Print and shaded views of the part. All mm, measured from the part's lowest x, y and z. A direction names the side the tool comes from. Round coordinates to 2 decimals unless told otherwise and drop trailing zeros. Write each loop counter-clockwise with the first axis right and the second up, starting at its lowest first coordinate (ties: lowest second). Pieces come first, ordered by that corner, then holes. Notation, with made-up numbers: M 64,7.5 L 115,7.5 A21 ccw 115,20.5 Z; hole C -19,13 d3. An arc over 180 degrees is marked long. Write item = value, one per line.
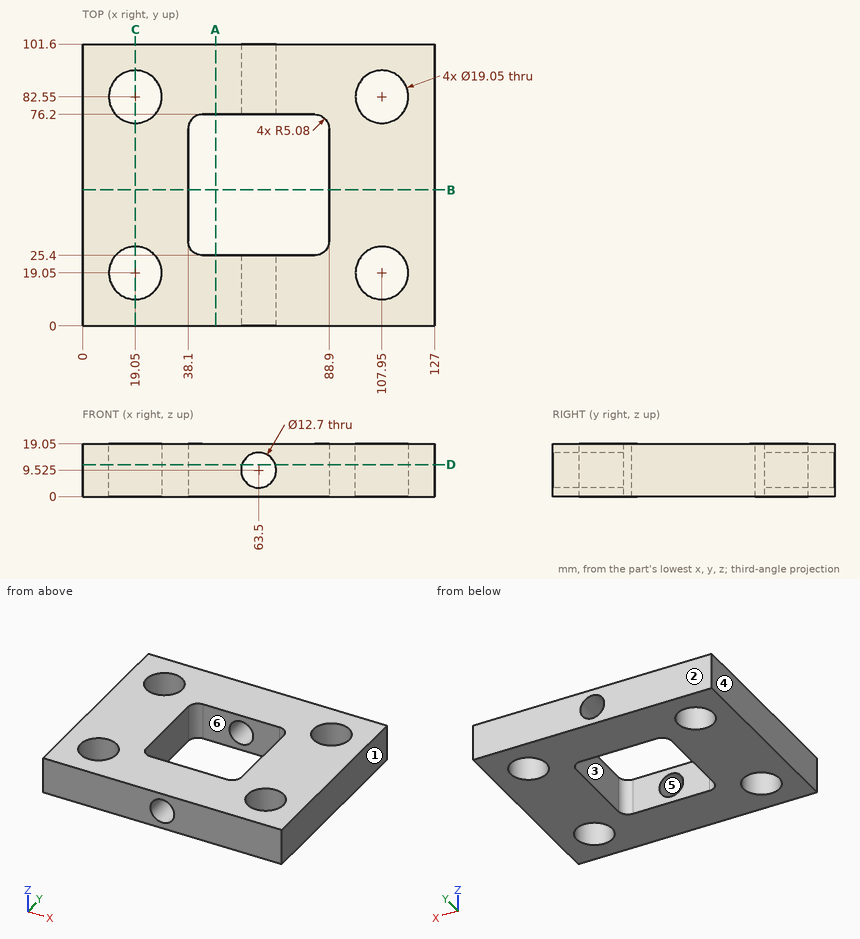
1. Flat gauge pin, fed straight in: pin 1 (17 mm diameter, centred on x = 107.95, y = 19.05, fed in from -Z). Where does the tip first touch, or does it go through?
Responses:
pin_1 = through
2. Band-saw the part on D-D (z = 11.5). List the corners of the cut face in (x, y) (3 decimals).
Responses:
outline = M 0,0 L 57.465,0 L 57.465,25.4 L 43.18,25.4 A5.08 cw 38.1,30.48 L 38.1,71.12 A5.08 cw 43.18,76.2 L 57.465,76.2 L 57.465,101.6 L 0,101.6 Z; M 69.535,0 L 127,0 L 127,101.6 L 69.535,101.6 L 69.535,76.2 L 83.82,76.2 A5.08 cw 88.9,71.12 L 88.9,30.48 A5.08 cw 83.82,25.4 L 69.535,25.4 Z; hole C 19.05,19.05 d19.05; hole C 19.05,82.55 d19.05; hole C 107.95,19.05 d19.05; hole C 107.95,82.55 d19.05
3. Mould opens along X. For the marked faces 1, 2, 3 and 4 say: pulls with the +X half, pulls with the -X half, needs draft (parallel to the pull), parting line crosses it, or undercut.
Responses:
face_1 = pulls with the +X half
face_2 = needs draft
face_3 = undercut
face_4 = pulls with the -X half
4. Band-saw the part on C-C (x = 19.05). List the corners of the cut face in (y, z) (3 decimals).
Responses:
outline = M 0,0 L 9.525,0 L 9.525,19.05 L 0,19.05 Z; M 28.575,0 L 73.025,0 L 73.025,19.05 L 28.575,19.05 Z; M 92.075,0 L 101.6,0 L 101.6,19.05 L 92.075,19.05 Z
5. Probe probe 1 along Y at (x, z) = (19.05, 4.75) (3 decimals); probe 2 along Y at (x, z) = (25, 7.5); probe 3 along X at (y, z) = (31.5, 9.75). List the from-to ranges inside material, lowest first.
Responses:
probe_1 = 0 to 9.525, 28.575 to 73.025, 92.075 to 101.6
probe_2 = 0 to 11.61, 26.49 to 75.11, 89.99 to 101.6
probe_3 = 0 to 38.1, 88.9 to 127
6. Tool access for the marked faces 5 and 6: list every direction of +Z, -Z, +X, -X, +Y, -Y with a clear straight run to the whole face (end or side of a thin tool).
Responses:
face_5 = +Y, -Y
face_6 = +Z, -Z
7. Band-saw the part on B-B (y = 49). List the corners of the cut face in (x, z).
Responses:
outline = M 0,0 L 38.1,0 L 38.1,19.05 L 0,19.05 Z; M 88.9,0 L 127,0 L 127,19.05 L 88.9,19.05 Z
8. Band-saw the part on A-A (x = 48). List the corners of the cut face in (y, z).
Responses:
outline = M 0,0 L 25.4,0 L 25.4,19.05 L 0,19.05 Z; M 76.2,0 L 101.6,0 L 101.6,19.05 L 76.2,19.05 Z
